Geometry check sheet. Reference: the model listing, model coordinates, mm. Face numbers are marked on the shaded views. A direction names the side the tool comes from. Give positions to 0.01 mm unless a question says otherwise; leave off trailing zeros. Order: outer loops, then holes, each group sorted by start corner. A loop starts at its lowest first (then second) coordinate and runs counter-clockwise, first axis right, second up. Notation, with made-up numbers: M 11,-20.75 L 19,-20.75 A16 cw 19,-16.75 Z; hole C 0.5,74 d8. An arc over 180 degrees is marked long. Answer as a JSON object with one key per item and string values. Group by question number.
from build123d import *

# Parameters (mm, degrees)
FILLET1_R          = 20
FILLET2_R          = 10
SKETCH2_R          = 4
CUT_EXTRUDE1_DEPTH = 120.824873174


with BuildPart() as part:
    # Sketch1 → Revolve1 (revolve)
    with BuildSketch(Plane(origin=(0, 0, 0), x_dir=(1, 0, 0), z_dir=(0, 1, 0)), mode=Mode.PRIVATE) as revolve1_sk:
        Polygon((0, -43), (-40, -43), (-40, -28), (-59, 28), (-59, 43), (0, 43), align=None)
    revolve(revolve1_sk.sketch.rotate(Axis((0, 0, 171.126428829), (0, 0, -1)), 180), axis=Axis((0, 0, 171.126428829), (0, 0, -1)))

    # Fillet1
    fillet1_edges = [part.edges().sort_by_distance(p)[0] for p in [
        (-59, 0, -28),
    ]]
    fillet(fillet1_edges, radius=FILLET1_R)

    # Fillet2
    fillet2_edges = [part.edges().sort_by_distance(p)[0] for p in [
        (-40, 0, 28),
    ]]
    fillet(fillet2_edges, radius=FILLET2_R)

    # Sketch2 → Cut-Extrude1 (cut, through all)
    with BuildSketch(Plane.XY.offset(43)):
        with Locations((0, 50)):
            Circle(SKETCH2_R)
        with Locations((50, 0)):
            Circle(SKETCH2_R)
        with Locations((0, -50)):
            Circle(SKETCH2_R)
        with Locations((-50, 0)):
            Circle(SKETCH2_R)
    extrude(amount=-CUT_EXTRUDE1_DEPTH, mode=Mode.SUBTRACT)


solid = part.part
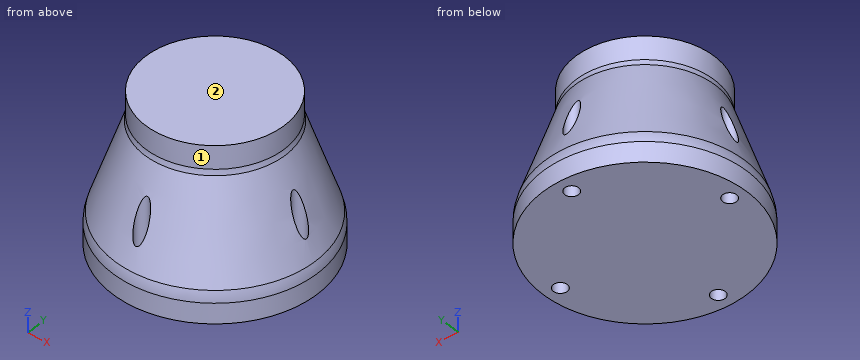
1. Cross-section at B-B (z = -5). Record the cut outline in (x, y), and give its area (3 significant figures).
2. Cross-section at D-D (z = 18.5). Record the cut outline in (x, y), and give its area (3 significant figures).
3. Thickness scan on line 1 along X through (y, z) = (1.5, -38); line 2 along Y through (x, z) = (0, -10); line 3 along X through (y, z) = (50, -17.5). Record the ranges inside material, lowest first. Write a range as [from, to].
4. Access from +Z, -Z, +X, -X, +Y, -Y to the whole of each face (thin tool, end or side, straight path). Record for the marked faces 1 and 2.
5. Cross-section at C-C (x = 0). State how many separate pieces and enclosed holes the cut face has, and give its area (3 significant figures).
6. Cross-section at A-A (z = -20.5). Record the cut outline in (x, y).
7. Depth check by flat-ended pin: pin 1 (8 mm diameter, centred on y = -20, z = 23, fed in from +X); pin 2 (5 mm diameter, centred on x = 39.5, z = -16, fed in from -Y); pin 3 (1 mm diameter, centred on y = 38, z = -9.5, fed in from -X). Enter the tip coordinate at first touch or a pass-through.
Report:
{
 "1": {"outline": "M -51.05,-3.86 A51.2 ccw -3.86,-51.05 A4 cw long 3.86,-51.05 A51.2 ccw 51.05,-3.86 A4 cw long 51.05,3.86 A51.2 ccw 3.86,51.05 A4 cw long -3.86,51.05 A51.2 ccw -51.05,3.86 A4 cw long Z", "area": "8,100 mm2"},
 "2": {"outline": "C 0,0 d86.45", "area": "5,870 mm2"},
 "3": {"line 1": "x = [-58.98, -53.71], [-46.29, 46.29], [53.71, 58.98]", "line 2": "y = [-46, 46]", "line 3": "x = [-23.94, -4], [4, 23.94]"},
 "4": {"face 1": "+Z", "face 2": "+Z, +X, -X, +Y, -Y"},
 "5": {"separate pieces": "3", "enclosed holes": "0", "area": "7,850 mm2"},
 "6": {"outline": "C 0,0 d112.91; hole C -50,0 d8; hole C 0,-50 d8; hole C 0,50 d8; hole C 50,0 d8"},
 "7": {"pin 1": "stops at x = 39.05", "pin 2": "stops at y = -40.87", "pin 3": "stops at x = -37.12"}
}
